Work out the finished part from the listing and answer in its coordinate system (mm). Face numbers are marked on the shaded views. Round coordinates to 2 decimals unless told otherwise and drop trailing zeros. Write each loop counter-clockwise with the first axis right and the second up, starting at its lowest first coordinate (ties: lowest second). Pieces come first, ordered by that corner, then holes. Notation, with made-up numbers: (70.5, 55.25) - (118.5, 55.25) arc R19 cw to (118.5, 72.25) - close; hole circle Ø4 at (0, -8.75). An arc over 180 degrees is marked (long way). Answer as a JSON object with one key per item and string values.
```python
from build123d import *

# Parameters (mm, degrees)
SKETCH1_R           = 1.5
BOSS_EXTRUDE1_DEPTH = 6
CHAMFER1_SIZE       = 0.5


with BuildPart() as part:
    # Sketch1 → Boss-Extrude1 (new, symmetric)
    with BuildSketch(Plane.XY):
        Polygon((3.464101615, 0), (1.732050808, 3), (-1.732050808, 3), (-3.464101615, 0), (-1.732050808, -3), (1.732050808, -3), align=None)
        Circle(SKETCH1_R, mode=Mode.SUBTRACT)
    extrude(amount=BOSS_EXTRUDE1_DEPTH, both=True)

    # Chamfer1
    chamfer1_edges = [part.edges().sort_by_distance(p)[0] for p in [
        (-1.5, 0, 6),
    ]]
    chamfer(chamfer1_edges, length=CHAMFER1_SIZE)


solid = part.part
```
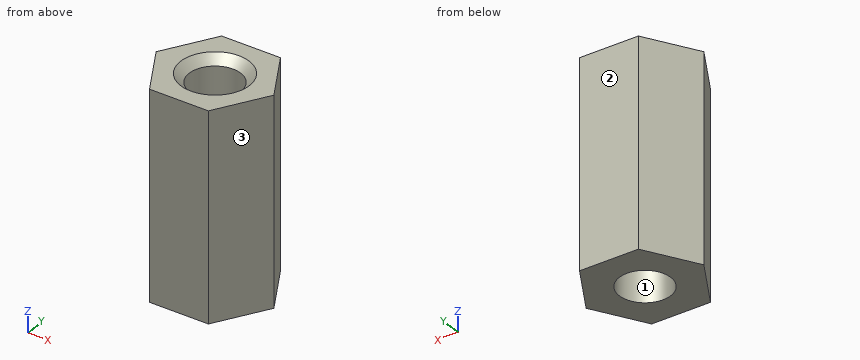
Item 1: Consider line 1 along Y through (x, z) = (0, -0.5); line 2 along Y through (x, z) = (-1.25, -3.25); line 3 along X through (y, z) = (1, -3.5). Determine where each line is inside the solid, lowest interval first.
Results found:
{"line 1": "-3 to -1.5, 1.5 to 3", "line 2": "-3 to -0.83, 0.83 to 3", "line 3": "-2.89 to -1.12, 1.12 to 2.89"}
Item 2: Determine the mould class of the marked faces 1, 2 and 3 for opening direction Y: pulls with the +Y half, pulls with the -Y half, needs draft (parallel to the pull), parting line crosses it, or undercut.
Results found:
{"face 1": "undercut", "face 2": "pulls with the +Y half", "face 3": "pulls with the -Y half"}
Item 3: A cutting plane is placed at D-D (y = 2.25). Write down the section's boundary in (x, z), and give its area (3 significant figures).
Results found:
{"outline": "(-2.17, -6) - (2.17, -6) - (2.17, 6) - (-2.17, 6) - close", "area": "52.0 mm²"}
Item 4: A cutting plane is placed at C-C (x = 2.25). Write down the section's boundary in (y, z), and give its area (3 significant figures).
Results found:
{"outline": "(-2.1, -6) - (2.1, -6) - (2.1, 6) - (-2.1, 6) - close", "area": "50.5 mm²"}
Item 5: A cutting plane is placed at A-A (x = 0). Write down the section's boundary in (y, z).
Results found:
{"outline": "(-3, -6) - (-1.5, -6) - (-1.5, 5.5) - (-2, 6) - (-3, 6) - close; (1.5, -6) - (3, -6) - (3, 6) - (2, 6) - (1.5, 5.5) - close"}
Item 6: A cutting plane is placed at B-B (z = -2.5). Write down the section's boundary in (x, y), and give its area (3 significant figures).
Results found:
{"outline": "(-3.46, 0) - (-1.73, -3) - (1.73, -3) - (3.46, 0) - (1.73, 3) - (-1.73, 3) - close; hole circle Ø3 at (0, 0)", "area": "24.1 mm²"}
